from build123d import *

# Parameters (mm, degrees)
CROQUIS1_W                    = 50
CROQUIS1_H                    = 40
SALIENTE_EXTRUIR1_DEPTH       = 12.5
TALADRO_DE_MARGEN_PARA_M81_D  = 8.4
TALADRO_DE_MARGEN_PARA_M161_D = 17


with BuildPart() as part:
    # Croquis1 → Saliente-Extruir1 (new body, symmetric)
    with BuildSketch(Plane.XY):
        Rectangle(CROQUIS1_W, CROQUIS1_H)
    extrude(amount=SALIENTE_EXTRUIR1_DEPTH, both=True)

    # Taladro de margen para M81 (through all)
    with Locations(Plane.XY.offset(12.5)):
        with Locations((-15, 10), (-15, -10), (15, -10), (15, 10)):
            Hole(TALADRO_DE_MARGEN_PARA_M81_D / 2)

    # Taladro de margen para M161 (through all)
    with Locations(Plane(origin=(0, 20, 0), x_dir=(1, 0, 0), z_dir=(0, 1, 0))):
        with Locations((0, 0)):
            Hole(TALADRO_DE_MARGEN_PARA_M161_D / 2)


solid = part.part
Part model, mm, in its own coordinate system. Coordinates: 2 decimals unless noted, no trailing zeros. Order: outer loops, then holes, each group sorted by start corner. A loop starts at its lowest first (then second) coordinate and runs counter-clockwise, first axis right, second up. Notation, with made-up numbers: (65, -32) - (117, -32) arc R17 cw to (117, -9) - close; hole circle Ø7 at (5, -22). An arc over 180 degrees is marked (long way). Use CSV: the item, a comma, the result in double quotes.
Item 1: Drop flat-ended pins along their axis: P1, Ø6.5, axis at x = 15, y = -10, coming from the +Z side; P2, Ø11, axis at x = -15, y = -10, coming from the -Z side. Give the stop position or say it passes through.
Solved:
P1,"passes through"
P2,"stops at z = -12.5"
Item 2: Mould opens along Y. For faces 1 (the face through (0, 20, 9)), 2 (the face through (0, -20, 9)), 3 (the face through (-11.904, 12.839, -0.175)) say: +Y half, -Y half, draft (parallel to the pull), parting line (faces both ways), or undercut.
Solved:
face 1,"+Y half"
face 2,"-Y half"
face 3,"undercut"
Item 3: Saw through at A-A on z = 0. Give the cut face in (x, y).
Solved:
outline,"(-25, -20) - (-8.5, -20) - (-8.5, 20) - (-25, 20) - close; (8.5, -20) - (25, -20) - (25, 20) - (8.5, 20) - close; hole circle Ø8.4 at (-15, -10); hole circle Ø8.4 at (-15, 10); hole circle Ø8.4 at (15, -10); hole circle Ø8.4 at (15, 10)"
Item 4: Saw through at C-C on y = 10. Give the cut face in (x, z).
Solved:
outline,"(-25, -12.5) - (-19.2, -12.5) - (-19.2, 12.5) - (-25, 12.5) - close; (-10.8, -12.5) - (10.8, -12.5) - (10.8, 12.5) - (-10.8, 12.5) - close; (19.2, -12.5) - (25, -12.5) - (25, 12.5) - (19.2, 12.5) - close; hole circle Ø17 at (0, 0)"
Item 5: Probe probe 1 along Y at (x, z) = (15, 0.25); probe 2 along Y at (x, z) = (12, 7.25); probe 3 along X at (y, z) = (6.5, -0.75). List the from-to ranges inside material, lowest first.
Solved:
probe 1,"y = -20 to -14.2, -5.8 to 5.8, 14.2 to 20"
probe 2,"y = -20 to -12.94, -7.06 to 7.06, 12.94 to 20"
probe 3,"x = -25 to -17.32, -12.68 to -8.47, 8.47 to 12.68, 17.32 to 25"
Item 6: Saw through at D-D on z = -9.5. Give the cut face in (x, y).
Solved:
outline,"(-25, -20) - (25, -20) - (25, 20) - (-25, 20) - close; hole circle Ø8.4 at (-15, -10); hole circle Ø8.4 at (-15, 10); hole circle Ø8.4 at (15, -10); hole circle Ø8.4 at (15, 10)"
Item 7: Saw through at B-B on x = -15. Give the cut face in (y, z), and give its area (3 significant figures).
Solved:
outline,"(-20, -12.5) - (-14.2, -12.5) - (-14.2, 12.5) - (-20, 12.5) - close; (-5.8, -12.5) - (5.8, -12.5) - (5.8, 12.5) - (-5.8, 12.5) - close; (14.2, -12.5) - (20, -12.5) - (20, 12.5) - (14.2, 12.5) - close"
area,"580 mm²"
